Autodesk Inventor part; units mm, degrees
ref_plane "YZ Plane" through (0, 0, 0) normal (1, 0, 0) x (0, 1, 0)
ref_plane "XZ Plane" through (0, 0, 0) normal (0, 1, 0) x (-1, 0, 0)
ref_plane "XY Plane" through (0, 0, 0) normal (0, 0, 1) x (1, 0, 0)
sketch "Sketch1" plane through (0, 0, 0) normal (0, 0, 1) x (1, 0, 0)
  line L0 (9.8795, 48.1994) -> (9.8795, -53.4006)
  line L1 (16.2295, 54.5494) -> (92.4295, 54.5494)
  line L2 (98.7795, 48.1994) -> (98.7795, -53.4006)
  line L3 (22.5795, -66.1006) -> (86.0795, -66.1006)
  arc A0 (9.8795, -53.4006) -> (22.5795, -66.1006) centre (22.5795, -53.4006) ccw
  arc A1 (16.2295, 54.5494) -> (9.8795, 48.1994) centre (16.2295, 48.1994) ccw
  arc A2 (98.7795, 48.1994) -> (92.4295, 54.5494) centre (92.4295, 48.1994) ccw
  arc A3 (86.0795, -66.1006) -> (98.7795, -53.4006) centre (86.0795, -53.4006) ccw
  point P0 (0, 0)
  dimension "d0" = 12.7
  dimension "d1" = 6.35
  dimension "d2" = 120.65
  dimension "d3" = 88.9
extrude "Extrusion1" add sketch "Sketch1" along normal blind 3.175
sketch "Sketch2" plane through (0, 0, 3.175) normal (0, 0, 1) x (1, 0, 0)
  line L0 (9.8795, -53.4006) -> (9.8795, 48.1994)
  line L1 (98.7795, 48.1994) -> (98.7795, -53.4006)
  line L2 (16.2295, 54.5494) -> (92.4295, 54.5494)
  line L3 (26.6435, 49.4694) -> (82.0155, 49.4694)
  line L4 (82.0155, 49.4694) -> (82.0155, -1.3306)
  line L5 (82.0155, -1.3306) -> (26.6435, -1.3306)
  line L6 (26.6435, -1.3306) -> (26.6435, 49.4694)
  point P0 (0, 0)
  dimension "d13" = 16.764
  dimension "d14" = 16.764
  dimension "d15" = 5.08
  dimension "d16" = 55.88
extrude "Extrusion2" cut sketch "Sketch2" against normal through all
sketch "Sketch3" plane through (0, 0, 3.175) normal (0, 0, 1) x (1, 0, 0)
  line L0 (9.8795, -53.4006) -> (9.8795, 48.1994)
  line L1 (86.0795, -66.1006) -> (22.5795, -66.1006)
  line L2 (9.8795, -19.4408) -> (32.7395, -19.4408)
  line L3 (32.7395, -19.4408) -> (32.7395, -37.2208)
  line L4 (32.7395, -37.2208) -> (9.8795, -37.2208)
  point P0 (0, 0)
  dimension "d20" = 28.8798
  dimension "d21" = 46.6598
  dimension "d22" = 22.86
extrude "Extrusion3" cut sketch "Sketch3" against normal through all
sketch "Sketch4" plane through (0, 0, 3.175) normal (0, 0, 1) x (1, 0, 0)
  line L0 (9.8795, -53.4006) -> (9.8795, -37.2208)
  arc A0 (9.8795, -53.4006) -> (22.5795, -66.1006) centre (22.5795, -53.4006) ccw
  line L1 (86.0795, -66.1006) -> (22.5795, -66.1006)
  line L2 (24.8655, -43.5708) -> (24.8655, -54.1626)
  line L3 (24.8655, -43.5708) -> (9.8795, -43.5708)
  line L4 (24.8655, -54.1626) -> (9.9024, -54.1626)
  point P0 (0, 0)
  dimension "d26" = 22.5298
  dimension "d27" = 14.986
  dimension "d28" = 11.938
extrude "Extrusion4" cut sketch "Sketch4" against normal through all
sketch "Sketch5" plane through (0, 0, 3.175) normal (0, 0, 1) x (1, 0, 0)
  line L0 (86.0795, -66.1006) -> (22.5795, -66.1006)
  line L1 (9.8795, -19.4408) -> (9.8795, 48.1994)
  line L2 (9.8795, -43.5708) -> (9.8795, -37.2208)
  line L3 (28.9295, -2.1688) -> (91.1595, -2.1688)
  line L4 (91.1595, -2.1688) -> (91.1595, -11.5668)
  line L5 (91.1595, -11.5668) -> (28.9295, -11.5668)
  line L6 (28.9295, -11.5668) -> (28.9295, -2.1688)
  line L7 (28.9295, -50.4288) -> (91.1595, -50.4288)
  line L8 (91.1595, -50.4288) -> (91.1595, -59.8268)
  line L9 (91.1595, -59.8268) -> (28.9295, -59.8268)
  line L10 (28.9295, -59.8268) -> (28.9295, -50.4288)
  point P0 (0, 0)
  dimension "d31" = 54.5338
  dimension "d32" = 9.398
  dimension "d33" = 62.23
  dimension "d34" = 19.05
  dimension "d35" = 19.05
  dimension "d36" = 6.2738
extrude "Extrusion5" cut sketch "Sketch5" against normal through all
sketch "Sketch8" plane through (0, 0, 3.175) normal (0, 0, 1) x (1, 0, 0)
  line L0 (91.1595, -11.5668) -> (28.9295, -11.5668)
  line L1 (28.9295, -50.4288) -> (91.1595, -50.4288)
  line L2 (91.1595, -50.4288) -> (91.1595, -59.8268)
  line L3 (9.8795, -43.5708) -> (24.8655, -43.5708)
  line L4 (24.8655, -43.5708) -> (24.8655, -54.1626)
  line L5 (86.0795, -66.1006) -> (22.5795, -66.1006)
  line L6 (98.7795, 48.1994) -> (98.7795, -53.4006)
  line L7 (9.8795, -19.4408) -> (9.8795, 48.1994)
  line L8 (9.8795, -19.4408) -> (32.7395, -19.4408)
  line L9 (32.7395, -37.2208) -> (9.8795, -37.2208)
  line L10 (9.8795, -43.5708) -> (9.8795, -37.2208)
  line L11 (96.2395, -11.5668) -> (96.2395, -32.3948)
  line L12 (96.2395, -32.3948) -> (98.7795, -32.3948)
  line L13 (91.1595, -11.5668) -> (96.2395, -11.5668)
  line L14 (98.7795, -50.1748) -> (91.1595, -50.1748)
  line L15 (9.8795, -3.4388) -> (27.1515, -3.4388)
  line L16 (27.1515, -3.4388) -> (27.1515, -19.4408)
  line L17 (34.0095, -11.5668) -> (34.0095, -38.3638)
  line L18 (31.2155, -38.3638) -> (31.2155, -50.4288)
  line L19 (30.0725, -37.2208) -> (30.0725, -45.4758)
  line L20 (24.8655, -45.4758) -> (30.0725, -45.4758)
  line L21 (31.2155, -38.3638) -> (34.0095, -38.3638)
  line L22 (91.1595, -50.4288) -> (91.1595, -50.1748)
  line L23 (12.4195, -3.4388) -> (12.4195, -19.4408)
  point P0 (0, 0)
  dimension "d63" = 2.54
  dimension "d67" = 15.9258
  dimension "d68" = 16.002
  dimension "d69" = 17.272
  dimension "d70" = 24.13
  dimension "d71" = 21.336
  dimension "d72" = 1.143
  dimension "d73" = 1.143
  dimension "d76" = 17.78
  dimension "d78" = 2.54
  dimension "d79" = 1.905
extrude "Extrusion11" cut sketch "Sketch8" against normal through all contours L13 L11 L12 L6 L14 L22 L1 L18 L21 L17 L0 | L10 L9 L19 L20 L4 L3 | L23 L15 L16 L8
sketch "Sketch9" plane through (0, 0, 3.175) normal (0, 0, 1) x (1, 0, 0)
  line L0 (98.7795, 48.1994) -> (98.7795, -32.3948)
  line L1 (16.2295, 54.5494) -> (92.4295, 54.5494)
  line L2 (9.8795, -19.4408) -> (9.8795, 48.1994)
  line L3 (86.0795, -66.1006) -> (22.5795, -66.1006)
  line L4 (36.2694, 49.7107) -> (34.2897, 49.7107)
  line L5 (34.2897, 49.7107) -> (33.2998, 51.4252)
  line L6 (33.2998, 51.4252) -> (34.2897, 53.1397)
  line L7 (34.2897, 53.1397) -> (36.2694, 53.1397)
  line L8 (36.2694, 53.1397) -> (37.2593, 51.4252)
  line L9 (37.2593, 51.4252) -> (36.2694, 49.7107)
  line L10 (14.7182, 34.5095) -> (13.0037, 33.5197)
  line L11 (13.0037, 33.5197) -> (11.2892, 34.5095)
  line L12 (11.2892, 34.5095) -> (11.2892, 36.4893)
  line L13 (11.2892, 36.4893) -> (13.0037, 37.4791)
  line L14 (13.0037, 37.4791) -> (14.7182, 36.4893)
  line L15 (14.7182, 36.4893) -> (14.7182, 34.5095)
  line L16 (14.7182, -3.5905) -> (13.0037, -4.5803)
  line L17 (13.0037, -4.5803) -> (11.2892, -3.5905)
  line L18 (11.2892, -3.5905) -> (11.2892, -1.6107)
  line L19 (11.2892, -1.6107) -> (13.0037, -0.6209)
  line L20 (13.0037, -0.6209) -> (14.7182, -1.6107)
  line L21 (14.7182, -1.6107) -> (14.7182, -3.5905)
  line L22 (75.3593, 51.4252) -> (74.3694, 49.7107)
  line L23 (74.3694, 49.7107) -> (72.3897, 49.7107)
  line L24 (72.3897, 49.7107) -> (71.3998, 51.4252)
  line L25 (71.3998, 51.4252) -> (72.3897, 53.1397)
  line L26 (72.3897, 53.1397) -> (74.3694, 53.1397)
  line L27 (74.3694, 53.1397) -> (75.3593, 51.4252)
  line L28 (97.3698, 34.5095) -> (95.6553, 33.5197)
  line L29 (95.6553, 33.5197) -> (93.9408, 34.5095)
  line L30 (93.9408, 34.5095) -> (93.9408, 36.4893)
  line L31 (93.9408, 36.4893) -> (95.6553, 37.4791)
  line L32 (95.6553, 37.4791) -> (97.3698, 36.4893)
  line L33 (97.3698, 36.4893) -> (97.3698, 34.5095)
  line L34 (95.6553, -4.5803) -> (93.9408, -3.5905)
  line L35 (93.9408, -3.5905) -> (93.9408, -1.6107)
  line L36 (93.9408, -1.6107) -> (95.6553, -0.6209)
  line L37 (95.6553, -0.6209) -> (97.3698, -1.6107)
  line L38 (97.3698, -1.6107) -> (97.3698, -3.5905)
  line L39 (97.3698, -3.5905) -> (95.6553, -4.5803)
  line L40 (36.2694, -64.6909) -> (34.2897, -64.6909)
  line L41 (34.2897, -64.6909) -> (33.2998, -62.9764)
  line L42 (33.2998, -62.9764) -> (34.2897, -61.2619)
  line L43 (34.2897, -61.2619) -> (36.2694, -61.2619)
  line L44 (36.2694, -61.2619) -> (37.2593, -62.9764)
  line L45 (37.2593, -62.9764) -> (36.2694, -64.6909)
  line L46 (75.3593, -62.9764) -> (74.3694, -64.6909)
  line L47 (74.3694, -64.6909) -> (72.3897, -64.6909)
  line L48 (72.3897, -64.6909) -> (71.3998, -62.9764)
  line L49 (71.3998, -62.9764) -> (72.3897, -61.2619)
  line L50 (72.3897, -61.2619) -> (74.3694, -61.2619)
  line L51 (74.3694, -61.2619) -> (75.3593, -62.9764)
  point P0 (0, 0)
  point P1 (35.2795, 51.4252)
  point P2 (13.0037, 35.4994)
  point P3 (13.0037, -2.6006)
  point P4 (73.3795, 51.4252)
  point P5 (95.6553, 35.4994)
  point P6 (95.6553, -2.6006)
  point P7 (35.2795, -62.9764)
  point P8 (73.3795, -62.9764)
  dimension "d80" = 3.1242
  dimension "d81" = 3.1242
  dimension "d82" = 38.1
  dimension "d83" = 3.429
  dimension "d84" = 19.05
  dimension "d85" = 25.4
  dimension "d86" = 38.1
  dimension "d87" = 3.1242
  dimension "d88" = 3.1242
extrude "Extrusion12" cut sketch "Sketch9" against normal through all
sketch "Sketch10" plane through (0, 0, 0) normal (0, 0, -1) x (-1, 0, 0)
  line L0 (-14.7182, -3.4388) -> (-14.7182, -1.6107)
  line L1 (-14.7182, -1.6107) -> (-13.0037, -0.6209)
  line L2 (-13.0037, -0.6209) -> (-11.2892, -1.6107)
  line L3 (-11.2892, -1.6107) -> (-11.2892, -3.5905)
  line L4 (-11.2892, -3.5905) -> (-12.4195, -4.243)
  line L5 (-12.4195, -4.243) -> (-12.4195, -19.4408)
  line L6 (-12.4195, -19.4408) -> (-9.8795, -19.4408)
  line L7 (-9.8795, 48.1994) -> (-9.8795, -19.4408)
  arc A0 (-9.8795, 48.1994) -> (-16.2295, 54.5494) centre (-16.2295, 48.1994) ccw
  line L8 (-92.4295, 54.5494) -> (-16.2295, 54.5494)
  arc A1 (-92.4295, 54.5494) -> (-98.7795, 48.1994) centre (-92.4295, 48.1994) ccw
  line L9 (-98.7795, -32.3948) -> (-98.7795, 48.1994)
  line L10 (-98.7795, -32.3948) -> (-96.2395, -32.3948)
  line L11 (-96.2395, -32.3948) -> (-96.2395, -11.5668)
  line L12 (-96.2395, -11.5668) -> (-91.1595, -11.5668)
  line L13 (-91.1595, -11.5668) -> (-91.1595, -2.1688)
  line L14 (-91.1595, -2.1688) -> (-28.9295, -2.1688)
  line L15 (-28.9295, -2.1688) -> (-28.9295, -11.5668)
  line L16 (-28.9295, -11.5668) -> (-34.0095, -11.5668)
  line L17 (-34.0095, -11.5668) -> (-34.0095, -38.3638)
  line L18 (-34.0095, -38.3638) -> (-31.2155, -38.3638)
  line L19 (-31.2155, -38.3638) -> (-31.2155, -50.4288)
  line L20 (-31.2155, -50.4288) -> (-28.9295, -50.4288)
  line L21 (-28.9295, -50.4288) -> (-28.9295, -59.8268)
  line L22 (-28.9295, -59.8268) -> (-91.1595, -59.8268)
  line L23 (-91.1595, -59.8268) -> (-91.1595, -50.1748)
  line L24 (-91.1595, -50.1748) -> (-98.7795, -50.1748)
  line L25 (-98.7795, -53.4006) -> (-98.7795, -50.1748)
  arc A2 (-98.7795, -53.4006) -> (-86.0795, -66.1006) centre (-86.0795, -53.4006) ccw
  line L26 (-22.5795, -66.1006) -> (-86.0795, -66.1006)
  arc A3 (-22.5795, -66.1006) -> (-9.9024, -54.1626) centre (-22.5795, -53.4006) ccw
  line L27 (-9.9024, -54.1626) -> (-24.8655, -54.1626)
  line L28 (-24.8655, -54.1626) -> (-24.8655, -45.4758)
  line L29 (-24.8655, -45.4758) -> (-30.0725, -45.4758)
  line L30 (-30.0725, -45.4758) -> (-30.0725, -37.2208)
  line L31 (-30.0725, -37.2208) -> (-32.7395, -37.2208)
  line L32 (-32.7395, -37.2208) -> (-32.7395, -19.4408)
  line L33 (-32.7395, -19.4408) -> (-27.1515, -19.4408)
  line L34 (-27.1515, -19.4408) -> (-27.1515, -3.4388)
  line L35 (-27.1515, -3.4388) -> (-14.7182, -3.4388)
  line L36 (-26.6435, 49.4694) -> (-26.6435, -1.3306)
  line L37 (-26.6435, -1.3306) -> (-82.0155, -1.3306)
  line L38 (-82.0155, -1.3306) -> (-82.0155, 49.4694)
  line L39 (-82.0155, 49.4694) -> (-26.6435, 49.4694)
  line L40 (-97.3698, 34.5095) -> (-97.3698, 36.4893)
  line L41 (-97.3698, 36.4893) -> (-95.6553, 37.4791)
  line L42 (-95.6553, 37.4791) -> (-93.9408, 36.4893)
  line L43 (-93.9408, 36.4893) -> (-93.9408, 34.5095)
  line L44 (-93.9408, 34.5095) -> (-95.6553, 33.5197)
  line L45 (-95.6553, 33.5197) -> (-97.3698, 34.5095)
  line L46 (-14.7182, 34.5095) -> (-14.7182, 36.4893)
  line L47 (-14.7182, 36.4893) -> (-13.0037, 37.4791)
  line L48 (-13.0037, 37.4791) -> (-11.2892, 36.4893)
  line L49 (-11.2892, 36.4893) -> (-11.2892, 34.5095)
  line L50 (-11.2892, 34.5095) -> (-13.0037, 33.5197)
  line L51 (-13.0037, 33.5197) -> (-14.7182, 34.5095)
  line L52 (-36.2694, -64.6909) -> (-37.2593, -62.9764)
  line L53 (-37.2593, -62.9764) -> (-36.2694, -61.2619)
  line L54 (-36.2694, -61.2619) -> (-34.2897, -61.2619)
  line L55 (-34.2897, -61.2619) -> (-33.2998, -62.9764)
  line L56 (-33.2998, -62.9764) -> (-34.2897, -64.6909)
  line L57 (-34.2897, -64.6909) -> (-36.2694, -64.6909)
  line L58 (-75.3593, 51.4252) -> (-74.3694, 53.1397)
  line L59 (-74.3694, 53.1397) -> (-72.3897, 53.1397)
  line L60 (-72.3897, 53.1397) -> (-71.3998, 51.4252)
  line L61 (-71.3998, 51.4252) -> (-72.3897, 49.7107)
  line L62 (-72.3897, 49.7107) -> (-74.3694, 49.7107)
  line L63 (-74.3694, 49.7107) -> (-75.3593, 51.4252)
  line L64 (-75.3593, -62.9764) -> (-74.3694, -61.2619)
  line L65 (-74.3694, -61.2619) -> (-72.3897, -61.2619)
  line L66 (-72.3897, -61.2619) -> (-71.3998, -62.9764)
  line L67 (-71.3998, -62.9764) -> (-72.3897, -64.6909)
  line L68 (-72.3897, -64.6909) -> (-74.3694, -64.6909)
  line L69 (-74.3694, -64.6909) -> (-75.3593, -62.9764)
  line L70 (-95.6553, -4.5803) -> (-97.3698, -3.5905)
  line L71 (-97.3698, -3.5905) -> (-97.3698, -1.6107)
  line L72 (-97.3698, -1.6107) -> (-95.6553, -0.6209)
  line L73 (-95.6553, -0.6209) -> (-93.9408, -1.6107)
  line L74 (-93.9408, -1.6107) -> (-93.9408, -3.5905)
  line L75 (-93.9408, -3.5905) -> (-95.6553, -4.5803)
  line L76 (-36.2694, 49.7107) -> (-37.2593, 51.4252)
  line L77 (-37.2593, 51.4252) -> (-36.2694, 53.1397)
  line L78 (-36.2694, 53.1397) -> (-34.2897, 53.1397)
  line L79 (-34.2897, 53.1397) -> (-33.2998, 51.4252)
  line L80 (-33.2998, 51.4252) -> (-34.2897, 49.7107)
  line L81 (-34.2897, 49.7107) -> (-36.2694, 49.7107)
  point P0 (0, 0)
  dimension "d91" = 16.764
  dimension "d92" = 72.136
  dimension "d93" = 115.57
  dimension "d94" = 64.77
equation "\"d14\" = d13"
equation "\"d35\" = d34"
equation "\"d73\" = d72"
properties part number "beagle_spacer_top"
Source: CAD feature listing. Evaluate the final solid. Frame: model axes, mm. A direction names the side the tool comes from. Give positions to 0.01 mm unless a question says otherwise; leave off trailing zeros. Write each loop counter-clockwise with the first axis right and the second up, starting at its lowest first coordinate (ties: lowest second). Pieces come first, ordered by that corner, then holes. Notation, with made-up numbers: M 27.5,78 L 84.5,78 A16 cw 84.5,109 Z; hole C 84.5,29.25 d1. An arc over 180 degrees is marked long. Return JSON: item names as keys, results as strings. Group by question number.
1) Pin query (flat end, axial travel): P1, Ø1.6, axis at y = -54, z = 1, coming from the +X side. Return the tip coordinate at first contact, or that it passes through.
2) Cut plane A-A, the plane y = -30. Output: boundary loops of the cut face in (x, z) (1 decimal).
3) Cut plane B-B, the plane x = 55. Output: boundary loops of the cut face in (y, z) (3 decimals).
4) Set-up query: faces 5 (the face through (97, -32.395, 2)), 6 (the face through (54, -66.101, 2)), 7 (the face through (28, -5, 0)), 8 (the face through (31, -37.221, 2)), 9 (the face through (91.16, -55, 2)). Return all of +Z, -Z, +X, -X, +Y, -Y with unobstructed straight access to the full face (end or side cutting, diameter ignored); none if empty.
5) Pull-direction query (X, two-part tool) for faces 1 (the face through (28.93, -7, 2)), 2 (the face through (12.42, -12, 2)), 3 (the face through (33, -38.364, 2)), 4 (the face through (13.971, -62.738, 1.565)); classes: pulls with the +X half, pulls with the -X half, needs draft (parallel to the pull), parting line crosses it, or undercut.
6) Cut plane D-D, the plane z = 1.1. Give the number of separate pieces and of enclosed holes in the cut face, plus the area to 3 significant figures.
7) Cut plane C-C, the plane x = 20. Output: boundary loops of the cut face in (y, z) (3 decimals).
8) Material intervals for line 1 along Y through (x, z) = (66, 2.4); line 2 along X through (y, z) = (-14, 2.7); line 3 along X through (y, z) = (44, 0.9), sorted ascending. Write a range as [from, to].
Recorded:
{
 "1": {"P1": "stops at x = 98.78"},
 "2": {"outline": "M 32.7,0 L 34,0 L 34,3.2 L 32.7,3.2 Z; M 96.2,0 L 98.8,0 L 98.8,3.2 L 96.2,3.2 Z"},
 "3": {"outline": "M -66.101,0 L -59.827,0 L -59.827,3.175 L -66.101,3.175 Z; M -2.169,0 L -1.331,0 L -1.331,3.175 L -2.169,3.175 Z; M 49.469,0 L 54.549,0 L 54.549,3.175 L 49.469,3.175 Z"},
 "4": {"face 5": "+Z, -Z, +X", "face 6": "+Z, -Z, +X, -X, -Y", "face 7": "-Z, +X, -X, +Y, -Y", "face 8": "+Z, -Z, -X", "face 9": "+Z, -Z"},
 "5": {"face 1": "undercut", "face 2": "undercut", "face 3": "needs draft", "face 4": "pulls with the -X half"},
 "6": {"separate pieces": "1", "enclosed holes": "8", "area": "3,140 mm²"},
 "7": {"outline": "M -65.836,0 L -54.163,0 L -54.163,3.175 L -65.836,3.175 Z; M -3.439,0 L 54.549,0 L 54.549,3.175 L -3.439,3.175 Z"},
 "8": {"line 1": "y = [-66.1, -59.83], [-2.17, -1.33], [49.47, 54.55]", "line 2": "x = [9.88, 12.42], [27.15, 34.01], [96.24, 98.78]", "line 3": "x = [9.88, 26.64], [82.02, 98.78]"}
}
